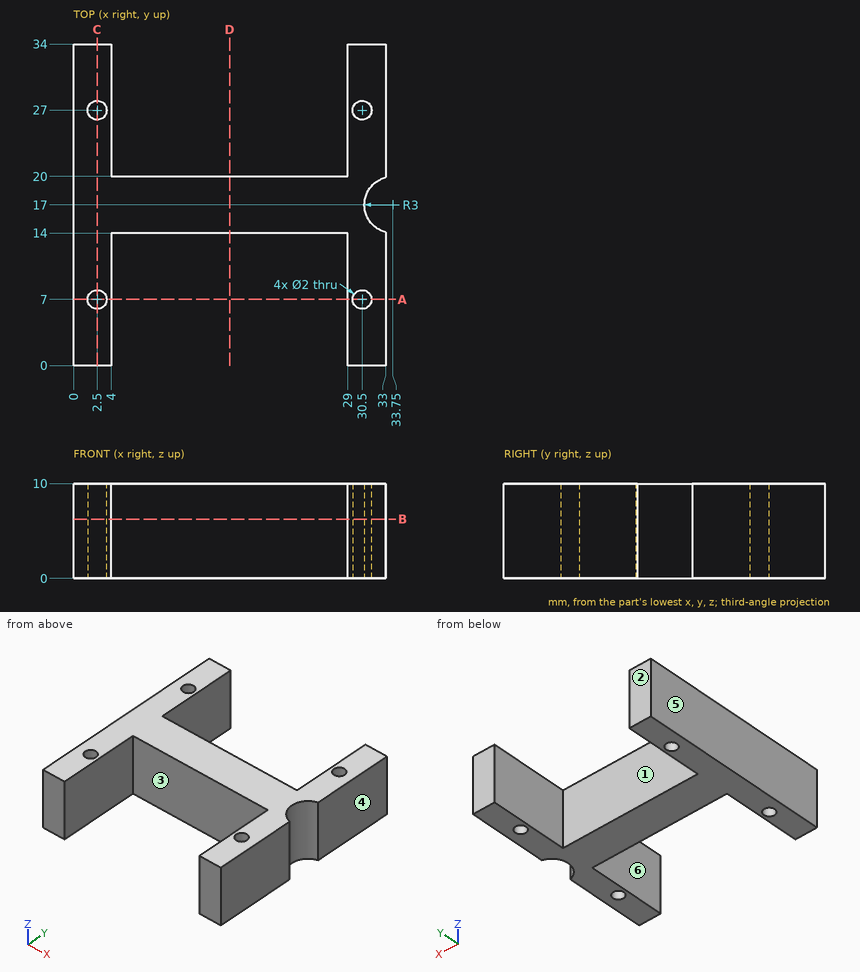
Geometry: see drawing. Coordinates: mm, zero at the bounding-box minimum. A direction names the side the tool comes from. Coordinates: 2 decimals unless noted, no trailing zeros. Loops run counter-clockwise (first coordinate to the right, second up) from the corner with the lowest first, then second, coordinate; pieces in that order, holes last. Notation, with made-up numbers: (63.25, 42.25) -> (116.25, 42.25) arc R16 ccw to (116.25, 63.25) -> close; hole circle Ø6 at (21.25, -22). An arc over 180 degrees is marked (long way). Write item = value, one per line. Start each with the question number.
Item 1: Cut plane B-B, the plane z = 6.25. Return loops of the section in (x, y), plus the area to 3 significant figures.
Item 2: Mould query, pull axis X, two halves, no side actions, for the marked faces 4, 5 and 6. Classes: pulls with the +X half, pulls with the -X half, needs draft (parallel to the pull), parting line crosses it, or undercut.
Item 3: Material intervals for line 1 (X direction, y = 27, z = 4.25); line 2 (Y direction, x = 2.5, z = 5); line 3 (X direction, y = 30, z = 3.25), sorted ascending.
Item 4: Reachability of the marked faces 1, 2 and 3 from +Z, -Z, +X, -X, +Y, -Y: full face, straight path, thin tool, end or side. Return the list, or none.
Item 5: Cut plane A-A, the plane y = 7. Return loops of the section in (x, z).
Item 6: Cut plane D-D, the plane x = 16.5. Return loops of the section in (y, z), plus the area to 3 significant figures.
Item 7: Cut plane C-C, the plane x = 2.5. Return loops of the section in (y, z), plus the area to 3 significant figures.
Item 8: First-contact query: P1, Ø1.5, axis at x = 12, z = 6.5, coming from the -Y side; P2, Ø1, axis at x = 18.5, z = 9, coming from the +Y side. Flat tips, straight axial feed; report the tip coordinate or a pass-through.
Ans:
q1.outline = (0, 0) -> (4, 0) -> (4, 14) -> (29, 14) -> (29, 0) -> (33, 0) -> (33, 14.1) arc R3 cw to (33, 19.9) -> (33, 34) -> (29, 34) -> (29, 20) -> (4, 20) -> (4, 34) -> (0, 34) -> close; hole circle Ø2 at (2.5, 7); hole circle Ø2 at (2.5, 27); hole circle Ø2 at (30.5, 7); hole circle Ø2 at (30.5, 27)
q1.area = 400 mm²
q2.face_4 = pulls with the +X half
q2.face_5 = pulls with the -X half
q2.face_6 = undercut
q3.line_1 = 0 to 1.5, 3.5 to 4, 29 to 29.5, 31.5 to 33
q3.line_2 = 0 to 6, 8 to 26, 28 to 34
q3.line_3 = 0 to 4, 29 to 33
q4.face_1 = +Z, -Z, +Y
q4.face_2 = +Z, -Z, +X, -X, +Y
q4.face_3 = +Z, -Z, -Y
q5.outline = (0, 0) -> (1.5, 0) -> (1.5, 10) -> (0, 10) -> close; (3.5, 0) -> (4, 0) -> (4, 10) -> (3.5, 10) -> close; (29, 0) -> (29.5, 0) -> (29.5, 10) -> (29, 10) -> close; (31.5, 0) -> (33, 0) -> (33, 10) -> (31.5, 10) -> close
q6.outline = (14, 0) -> (20, 0) -> (20, 10) -> (14, 10) -> close
q6.area = 60.0 mm²
q7.outline = (0, 0) -> (6, 0) -> (6, 10) -> (0, 10) -> close; (8, 0) -> (26, 0) -> (26, 10) -> (8, 10) -> close; (28, 0) -> (34, 0) -> (34, 10) -> (28, 10) -> close
q7.area = 300 mm²
q8.P1 = 14
q8.P2 = 20
